Read the model definition and answer for the solid it produces. Units are mm, in the model's axes. Face numbers are marked on the shaded views. A direction names the side the tool comes from. Coordinates: 2 decimals unless noted, no trailing zeros. Write each loop counter-clockwise with the first axis right and the second up, starting at its lowest first coordinate (ties: lowest second). Pieces come first, ordered by that corner, then holes. Notation, with made-up numbers: (1, 43.5) -> (30, 43.5) arc R7 ccw to (30, 49.5) -> close; hole circle Ø4 at (74, 2.5). An arc over 180 degrees is marked (long way). Return JSON: item names as keys, results as strings.
from build123d import *

# Parameters (mm, degrees)
SKETCH1_W                      = 88.9
SKETCH1_H                      = 88.9
SKETCH1_W_2                    = 82.55
SKETCH1_H_2                    = 82.55
BOSS_EXTRUDE1_DEPTH            = 762
CUT_EXTRUDE1_DEPTH             = 765.588520055
CUT_EXTRUDE1_DEPTH_BACK        = 765.588520055
SKETCH2_R                      = 4.2164
CUT_EXTRUDE2_DEPTH             = 769.45495151
CUT_EXTRUDE2_DEPTH_BACK        = 769.45495151
SKETCH3_R                      = 8.1915
SKETCH3_R_2                    = 4.2164
CUT_EXTRUDE3_REACH             = 770.455
SKETCH4_R                      = 8.1915
CUT_EXTRUDE3_DIRECTION_2_DEPTH = 769.45495151
F_3_8_CLEARANCE_HOLE2_D        = 9.8044
SKETCH10_R                     = 7.9375
CUT_EXTRUDE4_DEPTH             = 8.128
F_1_4_CLEARANCE_HOLE1_D        = 6.5278


with BuildPart() as part:
    # Sketch1 → Boss-Extrude1 (new body)
    with BuildSketch(Plane(origin=(0, 0, 0), x_dir=(1, 0, 0), z_dir=(0, 1, 0))):
        Rectangle(SKETCH1_W, SKETCH1_H)
        Rectangle(SKETCH1_W_2, SKETCH1_H_2, mode=Mode.SUBTRACT)
    extrude(amount=BOSS_EXTRUDE1_DEPTH)

    # Sketch2 → Cut-Extrude1 (cut, two sides: drawn at the far end of the back side and taken through both)
    with BuildSketch(Plane.XY.offset(-CUT_EXTRUDE1_DEPTH_BACK)):
        with Locations((-28.575, 25.4)):
            Circle(SKETCH2_R)
        with Locations((28.575, 25.4)):
            Circle(SKETCH2_R)
    extrude(amount=CUT_EXTRUDE1_DEPTH + CUT_EXTRUDE1_DEPTH_BACK, mode=Mode.SUBTRACT)

    # Sketch3 → Cut-Extrude2 (cut, two sides: drawn at the far end of the back side and taken through both)
    with BuildSketch(Plane.ZY.offset(44.45).offset(-CUT_EXTRUDE2_DEPTH_BACK)):
        with Locations((0, -13.00951767)):
            Circle(SKETCH3_R)
        with Locations((12.7, 19.05)):
            Circle(SKETCH3_R_2)
        with Locations((-12.7, 19.05)):
            Circle(SKETCH3_R_2)
    extrude(amount=CUT_EXTRUDE2_DEPTH + CUT_EXTRUDE2_DEPTH_BACK, mode=Mode.SUBTRACT)

    # Sketch4 → Cut-Extrude3 (cut, up to next)
    with BuildSketch(Plane(origin=(0, 0, -44.45), x_dir=(-1, 0, 0), z_dir=(0, 0, -1)), mode=Mode.PRIVATE) as cut_extrude3_sk1:
        with Locations((0, -2.54)):
            Circle(SKETCH4_R)
    cut_extrude3_tool1 = extrude(cut_extrude3_sk1.sketch, amount=-CUT_EXTRUDE3_REACH, mode=Mode.PRIVATE) & part.part
    add(cut_extrude3_tool1.solids().sort_by_distance((0, -2.54, -44.45))[0], mode=Mode.SUBTRACT)

    # Sketch4 → Cut-Extrude3 direction 2 (cut)
    with BuildSketch(Plane(origin=(0, 0, -44.45), x_dir=(-1, 0, 0), z_dir=(0, 0, -1))):
        with Locations((0, -2.54)):
            Circle(SKETCH4_R)
    extrude(amount=CUT_EXTRUDE3_DIRECTION_2_DEPTH, mode=Mode.SUBTRACT)

    # 3/8 Clearance Hole2 (through all)
    with Locations(Plane(origin=(28.575, 50.8, -44.45), x_dir=(-1, 0, 0), z_dir=(0, 0, -1))):
        with Locations((0, 0), (57.15, 0), (57.15, 123.825), (0, 123.825)):
            Hole(F_3_8_CLEARANCE_HOLE2_D / 2)

    # Sketch10 → Cut-Extrude4 (cut)
    with BuildSketch(Plane(origin=(0, 0, -44.45), x_dir=(-1, 0, 0), z_dir=(0, 0, -1))):
        with Locations((0, 383.9845)):
            Circle(SKETCH10_R)
    extrude(amount=-CUT_EXTRUDE4_DEPTH, mode=Mode.SUBTRACT)

    # 1/4 Clearance Hole1 (through all)
    with Locations(Plane(origin=(0, 0, -44.45), x_dir=(-1, 0, 0), z_dir=(0, 0, -1))):
        with Locations((25.4, 753.11), (-25.4, 753.11)):
            Hole(F_1_4_CLEARANCE_HOLE1_D / 2)


solid = part.part
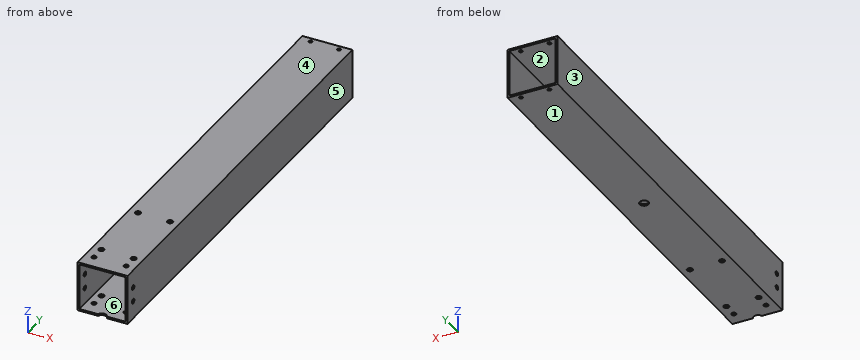
1. A tool of negligible diameter and unlimited length cuts with its end or side. For the marked faces 5 and 6, from which of +Z, -Z, +X, -X, +Y, -Y can it reach the whole face along a straight path? Write none if from no direction.
Taken from the geometry:
{"face 5": "+Z, -Z, +X, +Y, -Y", "face 6": "+Y, -Y"}
2. The part is cut by section A-A (x = 0). Count the separate pieces of the cut face and the enclosed holes in it, then the cut area to 3 significant figures.
Taken from the geometry:
{"separate pieces": "3", "enclosed holes": "0", "area": "4,770 mm2"}
3. For a pull along Z with two mould halves and no side action, classify the marked faces 1, 2, 3 and 4 as +Z half, -Z half, draft (parallel to the pull), parting line (faces both ways), or undercut.
Taken from the geometry:
{"face 1": "-Z half", "face 2": "undercut", "face 3": "draft", "face 4": "+Z half"}
4. The part is cut by section B-B (z = 32). Determine the outline of the cut face in (x, y) (3 decimals), then the cut area to 3 significant figures.
Taken from the geometry:
{"outline": "(-44.45, 0) -> (-41.275, 0) -> (-41.275, 762) -> (-44.45, 762) -> close; (41.275, 0) -> (44.45, 0) -> (44.45, 762) -> (41.275, 762) -> close", "area": "4,840 mm2"}
5. The part is cut by section C-C (y = 66). Determine the outline of the cut face in (x, z) (3 decimals), then the cut area to 3 significant figures.
Taken from the geometry:
{"outline": "(-44.45, -44.45) -> (44.45, -44.45) -> (44.45, 44.45) -> (-44.45, 44.45) -> close; hole (-41.275, -41.275) -> (41.275, -41.275) -> (41.275, 41.275) -> (-41.275, 41.275) -> close", "area": "1,090 mm2"}
6. Consider L1, parallel to Z at x = 42.7, y = 19.05; L2, parallel to X at y = 50, z = -43; L3, parallel to X at y = 25, z = 43. Determine where each line is inside the solid, lowest interval first.
Taken from the geometry:
{"L1": "z = -44.45 to -16.92, -8.48 to 8.48, 16.92 to 44.45", "L2": "x = -44.45 to -33.41, -23.74 to 23.74, 33.41 to 44.45", "L3": "x = -44.45 to -32.77, -24.38 to 24.38, 32.77 to 44.45"}
